```python
from build123d import *

# Parameters (mm, degrees)
F0_R     = 15.875
F1_DEPTH = 25.4
F2_R     = 5.08
F3_R     = 3.175
F4_DEPTH = 6.35
F5_R     = 2.54


with BuildPart() as f1:
    # F0 (on Front) → F1 (new body)
    with BuildSketch(Plane.XZ):
        Circle(F0_R)
    extrude(amount=F1_DEPTH)

    # F2
    f2_edges = [f1.edges().sort_by_distance(p)[0] for p in [
        (-15.875, -25.4, 0),
    ]]
    fillet(f2_edges, radius=F2_R)

    # F3 (on face) → F4 (join)
    with BuildSketch(Plane.XZ.offset(25.4)):
        Circle(F3_R)
    extrude(amount=F4_DEPTH)

    # F5
    f5_edges = [f1.edges().sort_by_distance(p)[0] for p in [
        (-3.175, -31.75, 0),
        (-3.175, -25.4, 0),
    ]]
    fillet(f5_edges, radius=F5_R)


solid = f1.part
```
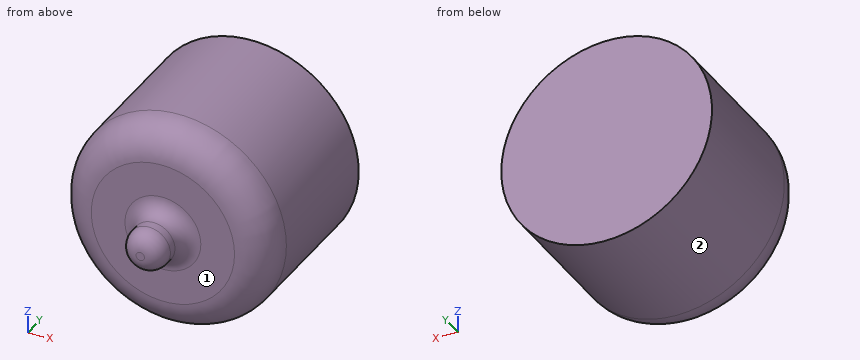
The listing builds one solid part. Answer for the finished solid, in the listing's coordinates (mm). Face numbers are marked on the shaded views. A direction names the side the tool comes from. Coordinates: 2 decimals unless noted, no trailing zeros. Loops run counter-clockwise (first coordinate to the right, second up) from the corner with the lowest first, then second, coordinate; pieces in that order, holes last. Notation, with made-up numbers: M 43.25,72.5 L 91.25,72.5 A26 cw 91.25,91.5 Z; hole C 32.5,44.5 d10. An arc over 180 degrees is marked long. Answer as CSV lines item,"result". Start each with the question number.
(1) For the marked faces 1 and 2, determine the directions among +Z, -Z, +X, -X, +Y, -Y from which every point of the face is accessible in a straight line to the end or side of a thin tool.
(2) The part is cut by section A-A (y = -16). Give the vertices of the cut face in (x, z) (3 decimals).
(3) Find the intervals of material crossed by L1, parallel to Y at x = 3.5, z = -7; L2, parallel to Z at x = -9, y = -23; L3, parallel to Z at x = 1.5, y = -14.5, in increasing order. Write a range as [from, to].
(4) Given pin 1 (2 mm diameter, centred on y = -13.5, z = 2, fed in from +X); pin 2 (1.5 mm diameter, centred on y = -25, z = 7.5, fed in from -X); pin 3 (1.5 mm diameter, centred on x = 8.5, z = -9, fed in from -Y), each flat-ended and moving along its own axis, determine where each tip first touches the part or whether it passes through.
Determined:
1,face 1,"-Y"
1,face 2,"+Y, -Y"
2,outline,"C 0,0 d31.75"
3,L1,"[-25.4, 0]"
3,L2,"[-12.14, 12.14]"
3,L3,"[-15.8, 15.8]"
4,pin 1,"x = 15.84"
4,pin 2,"x = -11.93"
4,pin 3,"y = -25.33"
